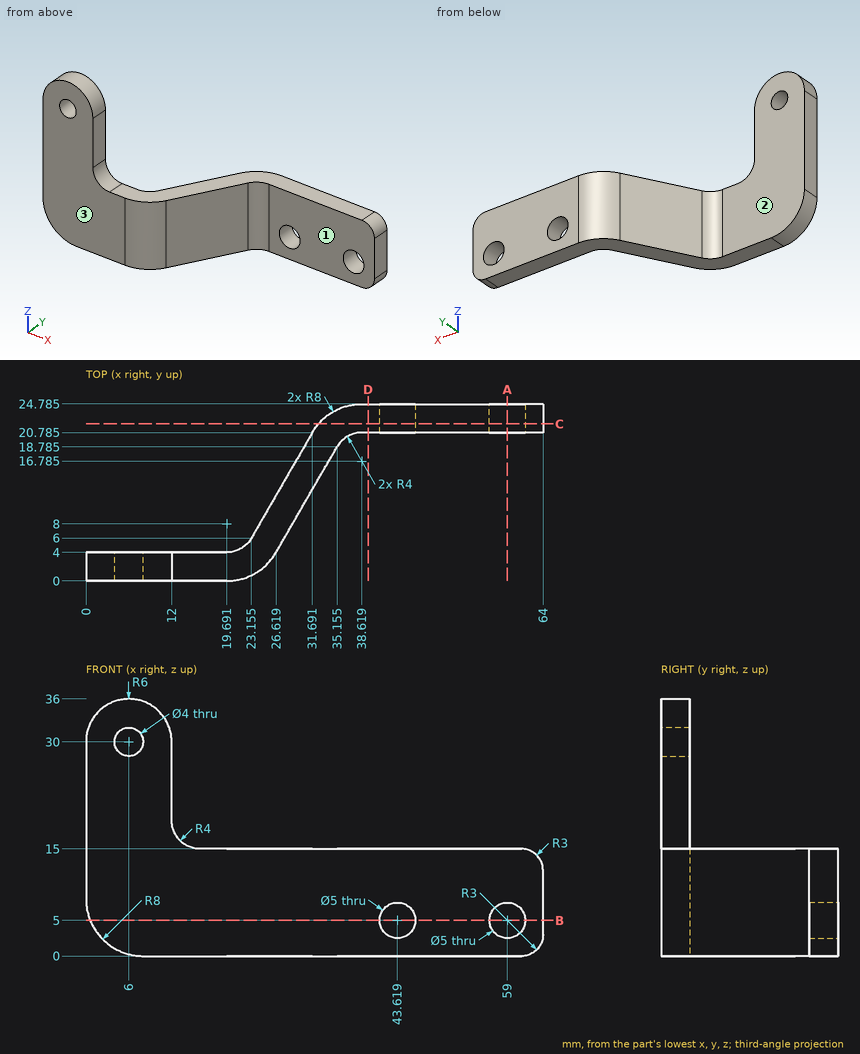
Geometry: see drawing. Coordinates: mm, zero at the bounding-box minimum. A direction names the side the tool comes from. Give positions to 0.01 mm unless a question says otherwise; leave off trailing zeros. Order: outer loops, then holes, each group sorted by start corner. A loop starts at its lowest first (then second) coordinate and runs counter-clockwise, first axis right, second up.
Q1. Section B-B on z = 5. Output: boundary loops of the cut face in (x, y) (1 decimal).
Checked values:
outline: (0.6, 0) - (19.7, 0) arc R8 ccw to (26.6, 4) - (35.2, 18.8) arc R4 cw to (38.6, 20.8) - (41.1, 20.8) - (41.1, 24.8) - (38.6, 24.8) arc R8 ccw to (31.7, 20.8) - (23.2, 6) arc R4 cw to (19.7, 4) - (0.6, 4) - close; (46.1, 20.8) - (56.5, 20.8) - (56.5, 24.8) - (46.1, 24.8) - close; (61.5, 20.8) - (64, 20.8) - (64, 24.8) - (61.5, 24.8) - close
Q2. Set-up query: the marked faces 1, 2 and 3. Return all of +Z, -Z, +X, -X, +Y, -Y with unobstructed straight access to the full face (end or side cutting, diameter ignored); none if empty.
Checked values:
face 1: +Z, -Z, +X, -Y
face 2: +Z, -Z, -X, +Y
face 3: +Z, -Z, +X, -X, -Y
Q3. Contact query for flat-ended pins moving along their axis: pin 1 Ø1.2 at (y, z) = (2.5, 25) entering from +X; pin 2 Ø21.5 at (x, z) = (11.5, 26.5) entering from +Y; pin 3 Ø8 at (y, z) = (12.5, 7) entering from -X. Output: stop coordinate, or through.
Checked values:
pin 1: stops at x = 12
pin 2: stops at y = 4
pin 3: stops at x = 24.6
Q4. Section A-A on x = 59. Output: boundary loops of the cut face in (y, z) (1 decimal), and give its area (3 significant figures).
Checked values:
outline: (20.8, 0) - (24.8, 0) - (24.8, 2.5) - (20.8, 2.5) - close; (20.8, 7.5) - (24.8, 7.5) - (24.8, 15) - (20.8, 15) - close
area: 40.0 mm2
Q5. Ray query, probe 1 along X at (y, z) = (24, 5) (1 decimal); probe 2 along Z at (x, y) = (59, 22.4); probe 3 along X at (y, z) = (23, 5). Return the intervals inside material, ascending.
Checked values:
probe 1: x = 35.2 to 41.1, 46.1 to 56.5, 61.5 to 64
probe 2: z = 0 to 2.5, 7.5 to 15
probe 3: x = 33.58 to 41.12, 46.12 to 56.5, 61.5 to 64
Q6. Section D-D on x = 39.5. Output: boundary loops of the cut face in (y, z) (1 decimal).
Checked values:
outline: (20.8, 0) - (24.8, 0) - (24.8, 15) - (20.8, 15) - close
Q7. Section C-C on y = 22. Output: boundary loops of the cut face in (x, z).
Checked values:
outline: (32.55, 0) - (61, 0) arc R3 ccw to (64, 3) - (64, 12) arc R3 ccw to (61, 15) - (32.55, 15) - close; hole circle Ø5 at (43.62, 5); hole circle Ø5 at (59, 5)
